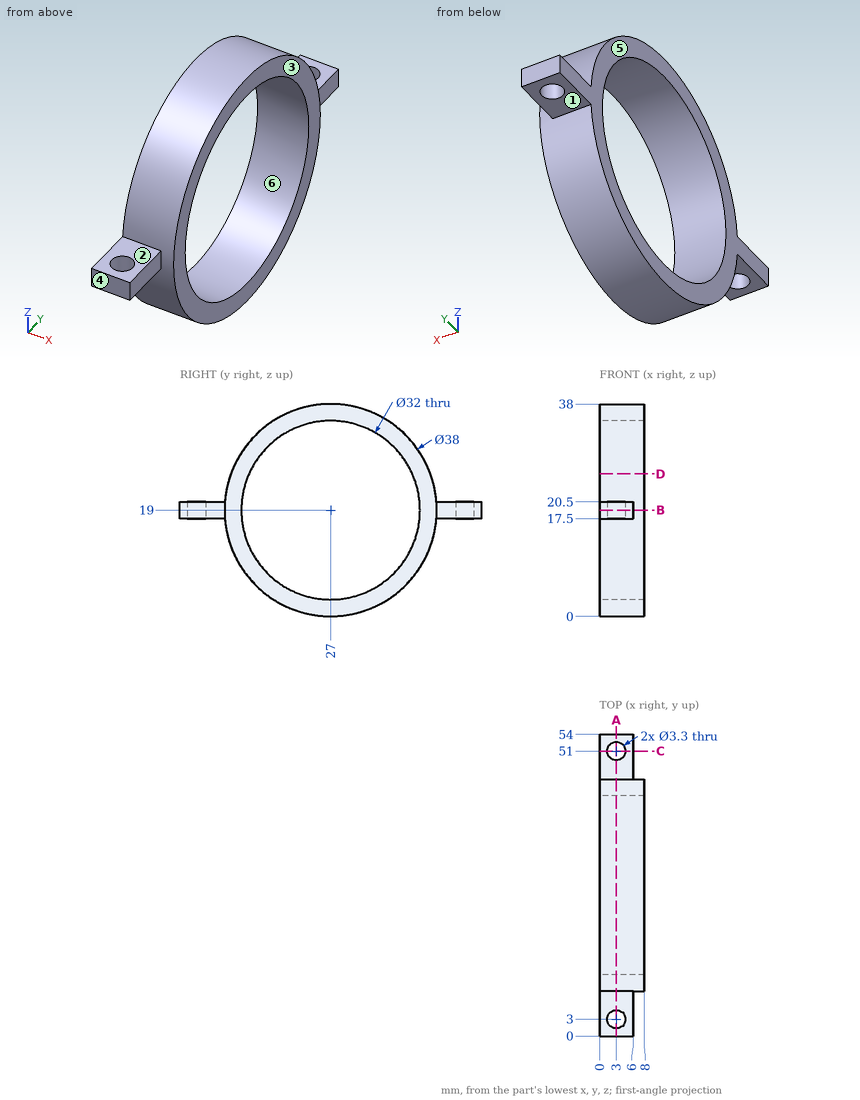
Design review of the part shown in the three views and the two pictorial views. Dimensions are in mm from the part's minimum x, y and z. A direction names the side the tool comes from. Round coordinates to 2 decimals unless told otherwise and drop trailing zeros. Write each loop counter-clockwise with the first axis right and the second up, starting at its lowest first coordinate (ties: lowest second). Pieces come first, ordered by that corner, then holes.
Item 1: Draft analysis for pull direction Y (two halves, no side actions). For the marked faces 4, 5 and 6, state which applies: released by +Y, released by -Y, zero draft, split by the parting line, or undercut.
Item 2: Consider section A-A on x = 3. Give the boundary of the cut face in (y, z).
Item 3: For pin 1 Ø1.5 at (x, z) = (5, 8) entering from +Y; pin 2 Ø2 at (x, y) = (6, 40) entering from -Z; pin 3 Ø4.5 at (x, y) = (3, 51) entering from +Z, all flat-tipped, find the tip position at first contact; note any pin that passes through.
Item 4: Consider section C-C on y = 51. Give the boundary of the cut face in (x, z).
Item 5: Consider section D-D on z = 25.5. Give the boundary of the cut face in (x, y), and give its area (3 significant figures).
Item 6: Wall thickness on L1, parallel to Y at x = 3, z = 19.3; L2, parallel to Z at x = 4, y = 27; L3, parallel to Y at x = 2.25, z = 28.5: over which ranges is each line inside the solid? List them lowest first.
Item 7: Consider section B-B on z = 19. Give the boundary of the cut face in (x, y), and give its area (3 significant figures).
Item 8: For the marked faces 1, 2 and 3, list the 3-axis set-ups (+Z, -Z, +X, -X, +Y, -Y) from which the entire face can be reached by the end or side of a thin tool; tool diameter is ignored.
Check values:
1. face 4: released by -Y
1. face 5: zero draft
1. face 6: undercut
2. outline: (0, 17.5) - (1.35, 17.5) - (1.35, 20.5) - (0, 20.5) - close; (4.65, 17.5) - (8.06, 17.5) arc R19 ccw to (45.94, 17.5) - (49.35, 17.5) - (49.35, 20.5) - (45.94, 20.5) arc R19 ccw to (8.06, 20.5) - (4.65, 20.5) - close; (52.65, 17.5) - (54, 17.5) - (54, 20.5) - (52.65, 20.5) - close; hole circle Ø32 at (27, 19)
3. pin 1: stops at y = 43
3. pin 2: stops at z = 4.27
3. pin 3: stops at z = 20.5
4. outline: (0, 17.5) - (1.35, 17.5) - (1.35, 20.5) - (0, 20.5) - close; (4.65, 17.5) - (6, 17.5) - (6, 20.5) - (4.65, 20.5) - close
5. outline: (0, 9.15) - (8, 9.15) - (8, 12.38) - (0, 12.38) - close; (0, 41.62) - (8, 41.62) - (8, 44.85) - (0, 44.85) - close
5. area: 51.7 mm2
6. L1: y = 0 to 1.35, 4.65 to 11, 43 to 49.35, 52.65 to 54
6. L2: z = 0 to 3, 35 to 38
6. L3: y = 10.55 to 14.13, 39.87 to 43.45
7. outline: (0, 0) - (6, 0) - (6, 8) - (8, 8) - (8, 11) - (0, 11) - close; (0, 43) - (8, 43) - (8, 46) - (6, 46) - (6, 54) - (0, 54) - close; hole circle Ø3.3 at (3, 3); hole circle Ø3.3 at (3, 51)
7. area: 127 mm2
8. face 1: -Z, +X, -X, +Y
8. face 2: +Z, +X, -X, -Y
8. face 3: +Z, -Z, +X, +Y, -Y
